CAD build for the part. Positions are in the model's coordinates, mm. A direction names the side the tool comes from. Coordinates: 2 decimals unless noted, no trailing zeros. Loops run counter-clockwise (first coordinate to the right, second up) from the corner with the lowest first, then second, coordinate; pieces in that order, holes last.
1) Which spindle directions (+Z, -Z, +X, -X, +Y, -Y) get a long thin tool onto all of the face, cutting with end or side? Do faces 4 (the flat face through (-37.88, 44, 15)), 5 (the cylindrical face through (-33.07, 5.03, 23.94)), 6 (the flat face through (2, 37.88, 15)), 7 (the flat face through (2, 3.98, 15)). Say none if no direction does.
2) Saw through at B-B, the plane x = -5.93. Write the cut outline in (y, z), and give its area (3 significant figures).
3) Saw through at D-D, the plane y = 26. Write the cut outline in (x, z).
4) Wall check: line 1 along Z through (x, y) = (-41.5, 16.5); line 2 along X through (y, z) = (19, 17.75); line 3 along X through (y, z) = (35.5, 26.25). Give the ranges that are in metal, low to high.
5) Two-plate mould, pull along Y, no slides. Class faces 1 (the cylindrical face through (-6.58, 38.86, 23.94)), 2 (the flat face through (-1.772, 1.833, 15.07)), 3 (the flat face through (4.12, 21, 15)): +Y half, -Y half, draft (parallel to the pull), parting line (faces both ways), or undercut.
6) Saw through at C-C, the plane z = 19.25. Write the cut outline in (x, y).
7) Saw through at A-A, the plane y = 5.93. Write the cut outline in (x, z), and give its area (3 significant figures).
8) Pin check, flat tips, straight feed: pin 1 Ø3 at (x, z) = (2.5, 14.5) entering from +Y; pin 2 Ø1.1 at (x, z) = (-44.5, 16.5) entering from -Y; pin 3 Ø6 at (x, y) = (-27, 6.5) entering from +Z. Stop position of each tip, or through.
Autodesk Inventor part; units mm, degrees
ref_plane "Work Plane2" through (-40.9959, 0.8639, 22.2359) normal (0, 0, 1) x (1, 0, 0)
ref_plane "YZ Plane" through (0, 0, 0) normal (1, 0, 0) x (0, 1, 0)
ref_plane "XZ Plane" through (0, 0, 0) normal (0, 1, 0) x (-1, 0, 0)
ref_plane "Work Plane1" through (0, 0, 10) normal (0, 0, 1) x (1, 0, 0)
sketch "Sketch1" plane through (0, 0, 10) normal (0, 0, 1) x (1, 0, 0)
  line L0 (-4.0299, -0.3538) -> (-2.2322, 1.4439) construction
  arc A0 (-1.4439, 2.2322) -> (-2.2322, 1.4439) centre (-0.9299, 0.9299) ccw construction
  line L1 (-1.4439, 2.2322) -> (0.3538, 4.0299) construction
  line L2 (-37.8299, 42.8299) -> (-37.8299, 37.8299) construction
  line L3 (-37.8299, 37.8299) -> (-42.9208, 37.8299) construction
  line L4 (-37.8299, 42.2137) -> (-37.8299, 45.8299) construction
  line L5 (-37.8299, 45.8299) -> (-4.0299, 45.8299) construction
  line L6 (-4.0299, 45.8299) -> (-4.0299, 42.2137) construction
  line L7 (-4.0299, 4.0299) -> (0.3538, 4.0299)
  circle A1 centre (-20.9299, 20.9299) radius 17.5
  line L8 (-20.9299, 58.9723) -> (17.1124, 20.9299) construction
  line L9 (17.1124, 20.9299) -> (-20.9299, -17.1124) construction
  line L10 (-20.9299, -17.1124) -> (-58.9723, 20.9299) construction
  line L11 (-58.9723, 20.9299) -> (-20.9299, 58.9723) construction
  line L12 (-20.9299, 58.9723) -> (-20.9299, -17.1124) construction
  line L13 (17.1124, 20.9299) -> (-58.9723, 20.9299) construction
  line L14 (-20.9299, 58.9723) -> (32.8701, 58.9723) construction
  line L15 (-43.4299, 43.4299) -> (1.5701, 43.4299) construction
  line L16 (1.5701, 43.4299) -> (1.5701, -1.5701) construction
  line L17 (1.5701, -1.5701) -> (-43.4299, -1.5701) construction
  line L18 (-43.4299, -1.5701) -> (-43.4299, 43.4299) construction
  line L19 (-43.4299, 43.4299) -> (1.5701, -1.5701) construction
  line L20 (1.5701, 43.4299) -> (-43.4299, -1.5701) construction
  line L21 (-43.4299, 5.3876) -> (-43.4299, 36.4723)
  line L22 (-43.4299, 36.4723) -> (-36.4723, 43.4299)
  line L23 (-36.4723, 43.4299) -> (-5.3876, 43.4299)
  line L24 (-5.3876, 43.4299) -> (1.5701, 36.4723)
  line L25 (1.5701, 36.4723) -> (1.5701, 5.3876)
  line L26 (1.5701, 5.3876) -> (-5.3876, -1.5701)
  line L27 (-5.3876, -1.5701) -> (-36.4723, -1.5701)
  line L28 (-36.4723, -1.5701) -> (-43.4299, 5.3876)
  line L29 (-4.0299, 42.2137) -> (-37.8299, 42.2137)
  line L30 (-4.0299, -0.3538) -> (-4.0299, 4.0299)
  point P0 (-37.8299, 4.0299)
  point P1 (-20.9299, 20.9299)
  dimension "d18" = 53.8
  dimension "d19" = 45
  dimension "d20" = 53.8
  dimension "d21" = 45
  dimension "d22" = 45
extrude "Extrusion1" add sketch "Sketch1" along normal blind 10
sketch "Sketch2" plane through (0, 0, 20) normal (0, 0, 1) x (1, 0, 0)
  circle A0 centre (-35.9299, 35.9299) radius 3.0099 construction
  circle A1 centre (-5.93, 35.9299) radius 3.0099 construction
  circle A2 centre (-5.93, 5.93) radius 3.0099 construction
  circle A3 centre (-35.9299, 5.93) radius 3.0099 construction
  circle A4 centre (-35.9299, 35.9299) radius 3
  circle A5 centre (-5.93, 35.9299) radius 3
  circle A6 centre (-5.93, 5.93) radius 3
  circle A7 centre (-35.9299, 5.93) radius 3
  point P0 (0, 0)
  dimension "d1" = 6
  dimension "d31" = 6
  dimension "d32" = 6
  dimension "d33" = 6
ref_plane "Work Plane2" through (-40.9959, 0.8639, 22.2359) normal (0, 0, 1) x (1, 0, 0)
extrude "Extrusion2" add sketch "Sketch2" along normal blind 8
sketch "Sketch3" plane through (0, 0, 10) normal (0, 0, -1) x (-1, 0, 0)
  line L0 (37.8299, -0.4701) -> (37.8299, 4.0299) construction
  line L1 (4.0299, 4.0299) -> (4.0299, -0.4701) construction
  line L2 (37.8299, -0.4701) -> (37.8299, 1.1886) construction
  line L3 (4.0299, -3.9701) -> (4.0299, -0.3538) construction
  line L4 (45.8299, 4.0299) -> (42.2137, 4.0299) construction
  line L5 (-0.3538, 4.0299) -> (-3.9701, 4.0299) construction
  line L6 (-3.9701, 37.8299) -> (-0.3538, 37.8299) construction
  line L7 (4.0299, 42.2137) -> (4.0299, 45.8299) construction
  line L8 (37.8299, 45.8299) -> (37.8299, 42.2137) construction
  line L9 (42.2137, 37.8299) -> (45.8299, 37.8299) construction
  line L10 (40.4657, 37.7299) -> (45.8299, 37.7299)
  line L11 (45.8299, 37.7299) -> (45.8299, 4.1299)
  line L12 (45.8299, 4.1299) -> (40.4657, 4.1299)
  line L13 (40.4657, 4.1299) -> (40.4657, 37.7299)
  line L14 (37.7299, 2.4952) -> (4.1299, 2.4952)
  line L15 (4.1299, 2.4952) -> (4.1299, -3.9701)
  line L16 (4.1299, -3.9701) -> (37.7299, -3.9701)
  line L17 (37.7299, -3.9701) -> (37.7299, 2.4952)
  line L18 (1.8946, 4.1299) -> (-3.9701, 4.1299)
  line L19 (-3.9701, 4.1299) -> (-3.9701, 37.7299)
  line L20 (-3.9701, 37.7299) -> (1.8946, 37.7299)
  line L21 (1.8946, 37.7299) -> (1.8946, 4.1299)
  line L22 (4.1299, 40.7326) -> (37.7299, 40.7326)
  line L23 (37.7299, 40.7326) -> (37.7299, 45.8299)
  line L24 (37.7299, 45.8299) -> (4.1299, 45.8299)
  line L25 (4.1299, 45.8299) -> (4.1299, 40.7326)
  point P0 (0, 0)
  dimension "d23" = 0.1
  dimension "d24" = 0.1
  dimension "d25" = 0.1
  dimension "d26" = 0.1
  dimension "d27" = 0.1
extrude "Extrusion3" add sketch "Sketch3" against normal up to surface (10 mm away)
sketch "Sketch4" plane through (0, 0, 20) normal (0, 0, 1) x (1, 0, 0)
  line L0 (3.9701, 4.1299) -> (0.3124, 4.1299)
  line L1 (3.9701, 37.7299) -> (3.9701, 4.1299)
  line L2 (0.3124, 37.7299) -> (3.9701, 37.7299)
  line L3 (0.3124, 37.7299) -> (-4.1299, 42.1723)
  line L4 (-4.1299, 45.8299) -> (-4.1299, 42.1723)
  line L5 (-37.7299, 45.8299) -> (-4.1299, 45.8299)
  line L6 (-37.7299, 42.1723) -> (-37.7299, 45.8299)
  line L7 (-37.7299, 42.1723) -> (-42.1723, 37.7299)
  line L8 (-45.8299, 37.7299) -> (-42.1723, 37.7299)
  line L9 (-45.8299, 4.1299) -> (-45.8299, 37.7299)
  line L10 (-42.1723, 4.1299) -> (-45.8299, 4.1299)
  line L11 (-42.1723, 4.1299) -> (-37.7299, -0.3124)
  line L12 (-37.7299, -3.9701) -> (-37.7299, -0.3124)
  line L13 (-4.1299, -3.9701) -> (-37.7299, -3.9701)
  line L14 (-4.1299, -0.3124) -> (-4.1299, -3.9701)
  line L15 (-4.1299, -0.3124) -> (0.3124, 4.1299)
  circle A0 centre (-20.9299, 20.9299) radius 17.5
  circle A1 centre (-35.9299, 5.93) radius 3
  circle A2 centre (-5.93, 35.9299) radius 3
  circle A3 centre (-35.9299, 35.9299) radius 3
  circle A4 centre (-5.93, 5.93) radius 3
  line L16 (-3.9799, 45.9799) -> (-3.9799, 42.2344)
  line L17 (-3.9799, 42.2344) -> (0.3745, 37.8799)
  line L18 (0.3745, 37.8799) -> (4.1201, 37.8799)
  line L19 (4.1201, 37.8799) -> (4.1201, 3.9799)
  line L20 (4.1201, 3.9799) -> (0.3745, 3.9799)
  line L21 (0.3745, 3.9799) -> (-3.9799, -0.3745)
  line L22 (-3.9799, -0.3745) -> (-3.9799, -4.1201)
  line L23 (-3.9799, -4.1201) -> (-37.8799, -4.1201)
  line L24 (-37.8799, -4.1201) -> (-37.8799, -0.3745)
  line L25 (-37.8799, -0.3745) -> (-42.2344, 3.9799)
  line L26 (-42.2344, 3.9799) -> (-45.9799, 3.9799)
  line L27 (-45.9799, 3.9799) -> (-45.9799, 37.8799)
  line L28 (-45.9799, 37.8799) -> (-42.2344, 37.8799)
  line L29 (-42.2344, 37.8799) -> (-37.8799, 42.2344)
  line L30 (-37.8799, 42.2344) -> (-37.8799, 45.9799)
  line L31 (-37.8799, 45.9799) -> (-3.9799, 45.9799)
  point P0 (0, 0)
  dimension "d34" = 0.15
extrude "Extrusion4" add sketch "Sketch4" against normal up to surface (10 mm away) contours L16 L17 L18 L19 L20 L21 L22 L23 L24 L25 L26 L27 L28 L29 L30 L31
ref_plane "Arbeitsebene3" through (-37.8799, 20.9299, 20) normal (0, -1, 0) x (1, 0, 0)
ref_plane "Arbeitsebene4" through (-20.9299, 3.9799, 20) normal (1, 0, 0) x (0, 0, -1)
equation "\"d31\" = d1"
equation "\"d32\" = d1"
equation "\"d33\" = d1"
properties part number "20_Cube_Insert_Thorlabs_Pins"
Data:
1. face 4: +Z, -Z, -X, +Y
1. face 5: +Z
1. face 6: +Z, -Z, +X, +Y
1. face 7: +Z, -Z, +X, -Y
2. outline: (-4.12, 10) - (11.92, 10) - (11.92, 20) - (8.93, 20) - (8.93, 28) - (2.93, 28) - (2.93, 20) - (-4.12, 20) - close; (29.94, 10) - (45.98, 10) - (45.98, 20) - (38.93, 20) - (38.93, 28) - (32.93, 28) - (32.93, 20) - (29.94, 20) - close
2. area: 417 mm2
3. outline: (-45.98, 10) - (-37.68, 10) - (-37.68, 20) - (-45.98, 20) - close; (-4.18, 10) - (4.12, 10) - (4.12, 20) - (-4.18, 20) - close
4. line 1: z = 10 to 20
4. line 2: x = -45.98 to -38.32, -3.54 to 4.12
4. line 3: x = -38.9 to -32.96, -8.9 to -2.96
5. face 1: undercut
5. face 2: -Y half
5. face 3: draft
6. outline: (-45.98, 3.98) - (-42.23, 3.98) - (-37.88, -0.37) - (-37.88, -4.12) - (-3.98, -4.12) - (-3.98, -0.37) - (0.37, 3.98) - (4.12, 3.98) - (4.12, 37.88) - (0.37, 37.88) - (-3.98, 42.23) - (-3.98, 45.98) - (-37.88, 45.98) - (-37.88, 42.23) - (-42.23, 37.88) - (-45.98, 37.88) - close; hole circle Ø35 at (-20.93, 20.93)
7. outline: (-45.98, 10) - (-29.94, 10) - (-29.94, 20) - (-32.93, 20) - (-32.93, 28) - (-38.93, 28) - (-38.93, 20) - (-45.98, 20) - close; (-11.92, 10) - (4.12, 10) - (4.12, 20) - (-2.93, 20) - (-2.93, 28) - (-8.93, 28) - (-8.93, 20) - (-11.92, 20) - close
7. area: 417 mm2
8. pin 1: stops at y = 37.88
8. pin 2: stops at y = 3.98
8. pin 3: stops at z = 20
